The listing builds one solid part. Answer for the finished solid, in the listing's coordinates (mm). Face numbers are marked on the shaded views. A direction names the side the tool comes from. Give positions to 0.01 mm unless a question says otherwise; leave off trailing zeros. Loops run counter-clockwise (first coordinate to the right, second up) from the corner with the lowest first, then second, coordinate; pieces in that order, holes last. Notation, with made-up numbers: (-3.75, 62.5) - (0.25, 62.5) arc R26 cw to (0.25, 76.5) - close; hole circle Ø11 at (28, -37). An arc over 180 degrees is marked (long way). Answer as CSV lines item,"result". Start each with the question number.
1) A cutting plane is placed at A-A (y = 0). Determine the outline of the cut face in (x, z) (3 decimals), and give its area (3 significant figures).
2) Flat-ended cylindrical pins translate along their axes: pin 1 (1 mm diameter, centred on x = -3.5, z = 9, fed in from -Y) (3 decimals); pin 2 (1.1 mm diameter, centred on y = 0.5, z = 13, fed in from -X); pin 3 (6 mm diameter, centred on y = 4.5, z = -7.5, fed in from -X). Find the tip coordinate at first contact, or state that the pin passes through.
3) Find the intervals of material crossed by line 1 along X through (y, z) = (-8, -6.5); line 2 along Y through (x, z) = (67.9, 0); line 3 along X through (y, z) = (7.25, -3.5), in increasing order.
4) For a pull along X with two mould halves and no side action, classify the marked faces 1, 2 and 3 as pulls with the +X half, pulls with the -X half, needs draft (parallel to the pull), parting line crosses it, or undercut.
5) A cutting plane is placed at B-B (x = 38.5). Determine the outline of the cut face in (y, z).
6) For the marked faces 4 and 5, determine the directions among +Z, -Z, +X, -X, +Y, -Y from which every point of the face is accessible in a straight line to the end or side of a thin tool.
7) A cutting plane is placed at C-C (y = 8.75). Determine the outline of the cut face in (x, z), and give its area (3 significant figures).
8) A cutting plane is placed at D-D (y = -8.5). Determine the outline of the cut face in (x, z).
```python
from build123d import *

# Parameters (mm, degrees)
F0_W     = 5.842
F0_H     = 12.7
F0_R     = 3.175
F2_DEPTH = 3.175
F3_R     = 1.524
F4_DEPTH = 3.81


with BuildPart() as f1:
    # F0 (on Front) → F1 (revolve)
    with BuildSketch(Plane.XZ):
        Polygon((5.842, 12.7), (5.842, 0), (66.294, 0), (66.294, 12.7), (56.134, 12.7), (56.134, 10.16), (10.16, 10.16), (10.16, 12.7), align=None)
        with Locations((2.921, 6.35)):
            Rectangle(F0_W, F0_H)
    revolve(axis=Axis((33.147, 0, 0), (-1, 0, 0)))

    # F0 (on Front) → F2 (join, symmetric)
    with BuildSketch(Plane.XZ):
        with Locations((2.921, 6.35)):
            Rectangle(F0_W, F0_H)
        with BuildLine():
            Line((-0.9398, 0), (0, 0))
            Line((0, 0), (0, 12.7))
            Line((0, 12.7), (5.842, 12.7))
            Line((5.842, 12.7), (5.842, 15.24))
            Line((5.842, 15.24), (-0.508, 15.24))
            Line((-0.508, 15.24), (-10.8806298187, 3.8475430269))
            ThreePointArc((-10.8806298187, 3.8475430269), (-4.5919612295, 5.3297205562), (-0.9398, 0))
        make_face()
        with BuildLine():
            Line((5.842, 0), (0, 0))
            Line((0, 0), (-0.9398, 0))
            ThreePointArc((-0.9398, 0), (-3.1957909266, -4.5493385486), (-8.1826630726, -5.5069827884))
            Line((-8.1826630726, -5.5069827884), (5.842, -9.398))
            Line((5.842, -9.398), (5.842, 0))
        make_face()
        with BuildLine():
            ThreePointArc((-8.1826630726, -5.5069827884), (-3.1957909266, -4.5493385486), (-0.9398, 0))
            ThreePointArc((-0.9398, 0), (-4.5919612295, 5.3297205562), (-10.8806298187, 3.8475430269))
            ThreePointArc((-10.8806298187, 3.8475430269), (-12.1459778134, -1.5837270034), (-8.1826630726, -5.5069827884))
        make_face()
        with Locations((-6.6548, 0)):
            Circle(F0_R, mode=Mode.SUBTRACT)
    extrude(amount=F2_DEPTH, both=True)

    # F3 (on face) → F4 (join, symmetric)
    with BuildSketch(Plane.YZ.offset(66.294)):
        with BuildLine():
            ThreePointArc((-5.08, 0), (0, 5.08), (5.08, 0))
            Line((5.08, 0), (5.08, 11.6397422652))
            ThreePointArc((5.08, 11.6397422652), (0, 12.7), (-5.08, 11.6397422652))
            Line((-5.08, 11.6397422652), (-5.08, 0))
        make_face()
        with BuildLine():
            ThreePointArc((-5.08, 0), (0, -5.08), (5.08, 0))
            ThreePointArc((5.08, 0), (0, 5.08), (-5.08, 0))
        make_face()
        Circle(F3_R, mode=Mode.SUBTRACT)
        with BuildLine():
            ThreePointArc((-5.08, 11.6397422652), (0, 12.7), (5.08, 11.6397422652))
            Line((5.08, 11.6397422652), (5.08, 15.24))
            Line((5.08, 15.24), (-5.08, 15.24))
            Line((-5.08, 15.24), (-5.08, 11.6397422652))
        make_face()
    extrude(amount=F4_DEPTH, both=True)


solid = f1.part
```
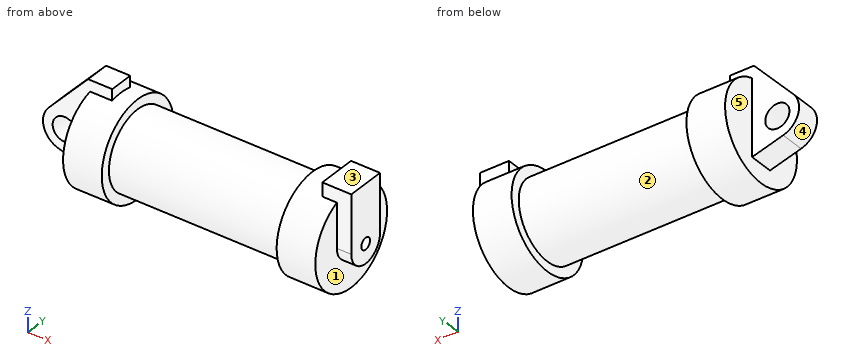
Ans:
1,outline,"(-10.881, 3.848) arc R5.715 ccw to (-8.183, -5.507) - (0, -7.777) - (0, -12.7) - (10.16, -12.7) - (10.16, -10.16) - (56.134, -10.16) - (56.134, -12.7) - (66.294, -12.7) - (66.294, -5.08) - (70.104, -5.08) - (70.104, -1.524) - (66.294, -1.524) - (66.294, 1.524) - (70.104, 1.524) - (70.104, 15.24) - (62.484, 15.24) - (62.484, 12.7) - (56.134, 12.7) - (56.134, 10.16) - (10.16, 10.16) - (10.16, 12.7) - (5.842, 12.7) - (5.842, 15.24) - (-0.508, 15.24) - close; hole circle Ø6.35 at (-6.655, 0)"
1,area,"1,690 mm2"
2,pin 1,"y = -3.175"
2,pin 2,"x = -3.05"
2,pin 3,"x = -9.74"
3,line 1,"0 to 10.16, 56.13 to 66.29"
3,line 2,"-5.08 to -1.52, 1.52 to 5.08"
3,line 3,"0 to 66.29"
4,face 1,"pulls with the +X half"
4,face 2,"undercut"
4,face 3,"needs draft"
5,outline,"circle Ø20.32 at (0, 0)"
6,face 4,"-X, +Y, -Y"
6,face 5,"-Z, -X"
7,outline,"(0, -9.2) - (10.16, -9.2) - (10.16, -5.16) - (56.13, -5.16) - (56.13, -9.2) - (66.29, -9.2) - (66.29, 9.2) - (56.13, 9.2) - (56.13, 5.16) - (10.16, 5.16) - (10.16, 9.2) - (0, 9.2) - close"
7,area,"849 mm2"
8,outline,"(0, -9.44) - (10.16, -9.44) - (10.16, -5.57) - (56.13, -5.57) - (56.13, -9.44) - (66.29, -9.44) - (66.29, 9.44) - (56.13, 9.44) - (56.13, 5.57) - (10.16, 5.57) - (10.16, 9.44) - (0, 9.44) - close"
